Can you work these out from the model? Positions are in its coordinate system, mm. A direction names the side the tool comes from. Give positions to 0.01 mm unless a question says otherwise; leave off trailing zeros. Order: outer loops, then holes, each group sorted by start corner. A loop starts at its lowest first (then second) coordinate and runs counter-clockwise, first axis right, second up. Notation, with made-up numbers: (60.25, -28) -> (89.25, -28) arc R15 ccw to (89.25, -1) -> close; hole circle Ø4 at (62.25, 39). An arc over 180 degrees is marked (long way). Answer as CSV lines item,"result".
```python
from build123d import *

# Parameters (mm, degrees)
F1_DEPTH    = 175
F2_T1_DEPTH = 875


# Not quite as in the source:
# - a fillet or chamfer that OpenCascade refuses, or shapes differently, is made with other operations: its cross-section is extruded or revolved along the edge and cut away or added


with BuildPart() as f1:
    # F0 (on Front) → F1 (new body, symmetric)
    with BuildSketch(Plane.XZ):
        with BuildLine():
            Line((-750, 0), (0, 0))
            Line((0, 0), (0, 5))
            Line((0, 5), (-750, 5))
            ThreePointArc((-750, 5), (-850.8959422811, 22.7906768682), (-939.6223448575, 74.0168892799))
            Line((-939.6223448575, 74.0168892799), (-942.836282906, 70.1866670643))
            ThreePointArc((-942.836282906, 70.1866670643), (-852.6060429977, 18.0922137642), (-750, 0))
        make_face()
    extrude(amount=F1_DEPTH, both=True)

    # F2: fillet of radius 174 on 2 edges, made by hand

    # F2_s2 → F2_t1 (cut)
    with BuildSketch(Plane(origin=(-72.170505067, 0, -86.0094586929), x_dir=(0, 1, 0), z_dir=(-0.6427876097, 0, -0.7660444431))):
        with BuildLine():
            ThreePointArc((-1, -767.3696152452), (-124.0365799265, -716.4061951717), (-175, -593.3696152452))
            Line((-175, -593.3696152452), (-175, -767.3696152452))
            Line((-175, -767.3696152452), (-1, -767.3696152452))
        make_face()
        with BuildLine():
            ThreePointArc((1, -767.3696152452), (124.0365799265, -716.4061951717), (175, -593.3696152452))
            Line((175, -593.3696152452), (175, -767.3696152452))
            Line((175, -767.3696152452), (1, -767.3696152452))
        make_face()
    extrude(amount=F2_T1_DEPTH, mode=Mode.SUBTRACT)

    # F3: F1 across plane


with BuildPart() as f1_1:
    add(f1.part)
    add(f1.part.mirror(Plane.YZ))


solid = f1_1.part
```
Item 1: Imagine slicing it at B-B, the plane x = 452. Please give me the cut outline in (y, z).
Numbers:
outline,"(-175, 0) -> (175, 0) -> (175, 5) -> (-175, 5) -> close"
Item 2: Please list where these lines run through material, in increasing order: line 1 along Z through (x, y) = (-267, 26.5); line 2 along Z through (x, y) = (757.5, 62.5); line 3 along X through (y, z) = (-88.5, 56).
Numbers:
line 1,"z = 0 to 5"
line 2,"z = 0.09 to 5.1"
line 3,"x = -923.93 to -915.8, 915.8 to 923.93"
Item 3: Imagine slicing it at A-A, the plane y = -81. Please give me the cut outline in (x, z).
Numbers:
outline,"(-927.51, 58.15) arc R300 ccw to (-750, 0) -> (750, 0) arc R300 ccw to (927.51, 58.15) -> (924.28, 61.99) arc R295 cw to (750, 5) -> (-750, 5) arc R295 cw to (-924.28, 61.99) -> close"
Item 4: For pin 1 (2 mm diameter, centred on x = -150.5, y = -119.5, fed in from +Z); pin 2 (1.5 mm diameter, centred on x = 37, z = 7.5, fed in from -Y) (3 decimals); pin 3 (4 mm diameter, centred on y = 111, z = 33.5, fed in from -X), each with a flat end and sliding along its axis, tell me the tip position at first contact or that it passes through.
Numbers:
pin 1,"stops at z = 5"
pin 2,"passes through"
pin 3,"stops at x = -891.56"
Item 5: For faces 4 (the cylindrical face through (898.9, -123.585, 43.963)), 5 (the cylindrical face through (-827.72, -2.45, 15.42)), which set-ups out of +Z, -Z, +X, -X, +Y, -Y let a thin tool reach every point of the face, with its end or its side?
Numbers:
face 4,"+Z, +X, -Y"
face 5,"+Z, +Y, -Y"
Item 6: We'd pull the mould along X, two halves only. Please class faces 1 (the cylindrical face through (831.863, -2.45, 11.385)), 2 (the cylindrical face through (-898.9, -123.585, 43.963)), 3 (the flat face through (-10, -2, 5)): released by +X, released by -X, zero draft, split by the parting line, or undercut.
Numbers:
face 1,"released by +X"
face 2,"released by -X"
face 3,"undercut"
Item 7: Imagine slicing it at C-C, the plane y = 21.5. Please give me the cut outline in (x, z).
Numbers:
outline,"(-941.91, 69.41) arc R300 ccw to (-750, 0) -> (750, 0) arc R300 ccw to (941.91, 69.41) -> (938.69, 73.24) arc R295 cw to (750, 5) -> (-750, 5) arc R295 cw to (-938.69, 73.24) -> close"
